Study the drawing (mm; zero at the part's minimum x, y, z) and answer. Round coordinates to 2 decimals unless told otherwise and drop trailing zeros. Write each loop counter-clockwise with the first axis right and the second up, starting at its lowest first coordinate (ties: lowest second). Pieces come first, ordered by that corner, then holes. Notation, with made-up numbers: (40.25, 14) - (44.25, 14) arc R15 ccw to (44.25, 32) - close; hole circle Ø7 at (-26, 12). An arc over 180 degrees is marked (long way). Use one line per item in the form item = value. Start each with the question number.
1) The part is cut by section B-B, the plane z = 34. Give the vertices of the cut face in (x, y), plus the area to 3 significant figures.
2) Consider line 1 along X through (y, z) = (2.85, 14); line 2 along X through (y, z) = (0.9, 6.5); line 3 along Z through (x, y) = (7, 2.4). Determine where each line is inside the solid, lowest interval first. Write a range as from..to.
3) The part is cut by section C-C, the plane y = 2.3. Give the vertices of the cut face in (x, z).
4) This flat-tipped pin is pushed along its axis until it touches: pin 1 (1.2 mm diameter, centred on x = 37.5, y = 3, fed in from -Z). Where does it stop, or does it pass through?
5) The part is cut by section A-A, the plane x = 50.5. Give the vertices of the cut face in (y, z), plus the area to 3 significant figures.
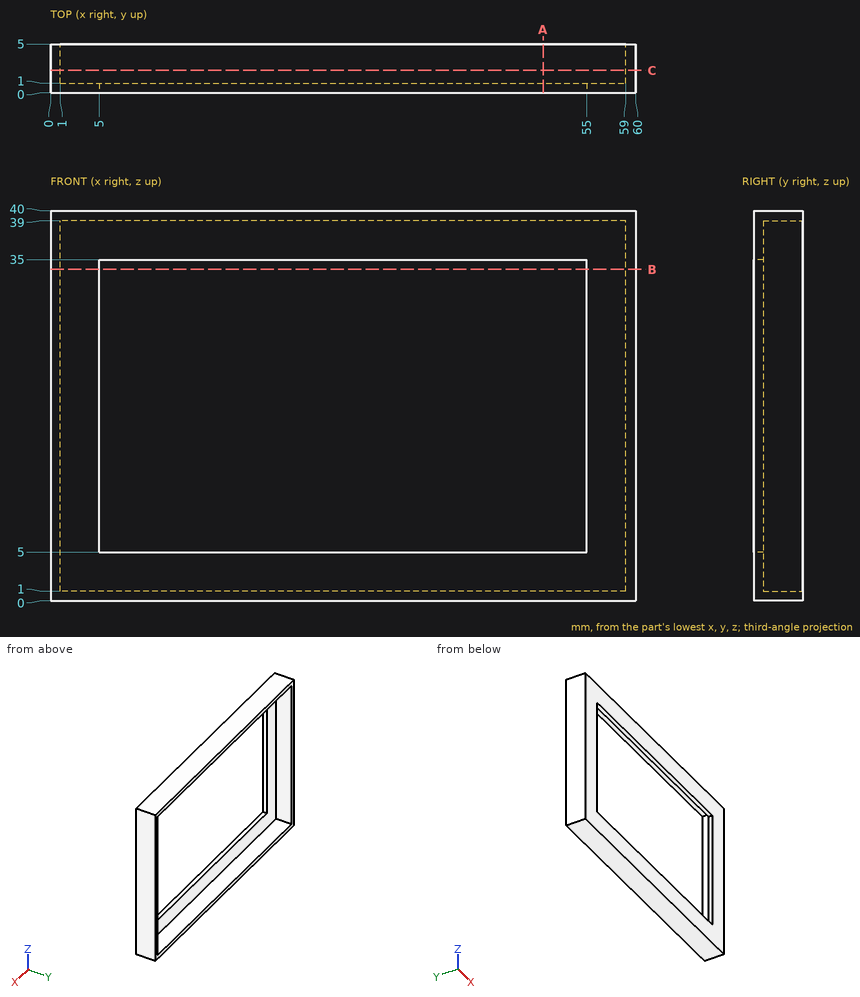
Geometry results:
q1.outline = (0, 0) - (5, 0) - (5, 1) - (1, 1) - (1, 5) - (0, 5) - close; (55, 0) - (60, 0) - (60, 5) - (59, 5) - (59, 1) - (55, 1) - close
q1.area = 18.0 mm2
q2.line_1 = 0..1, 59..60
q2.line_2 = 0..5, 55..60
q2.line_3 = 0..1, 39..40
q3.outline = (0, 0) - (60, 0) - (60, 40) - (0, 40) - close; hole (1, 1) - (59, 1) - (59, 39) - (1, 39) - close
q4.pin_1 = 0
q5.outline = (0, 0) - (5, 0) - (5, 1) - (1, 1) - (1, 5) - (0, 5) - close; (0, 35) - (1, 35) - (1, 39) - (5, 39) - (5, 40) - (0, 40) - close
q5.area = 18.0 mm2
